```python
from build123d import *

# Parameters (mm, degrees)
F0_W     = 31.75
F0_H     = 44.45
F0_R     = 1.5875
F1_DEPTH = 25.4
F2_R     = 1.1303
F3_DEPTH = 6.35


with BuildPart() as f1:
    # F0 (on Front) → F1 (new body)
    with BuildSketch(Plane.XZ):
        with Locations((-15.875, 22.225)):
            Rectangle(F0_W, F0_H)
        with Locations((-25.4, 25.4)):
            Circle(F0_R, mode=Mode.SUBTRACT)
    extrude(amount=F1_DEPTH)

    # F2 (on Top) → F3 (cut)
    with BuildSketch(Plane.XY):
        with Locations((-21.166667, -12.7)):
            Circle(F2_R)
        with Locations((-10.583333, -12.7)):
            Circle(F2_R)
    extrude(amount=F3_DEPTH, mode=Mode.SUBTRACT)


solid = f1.part
```
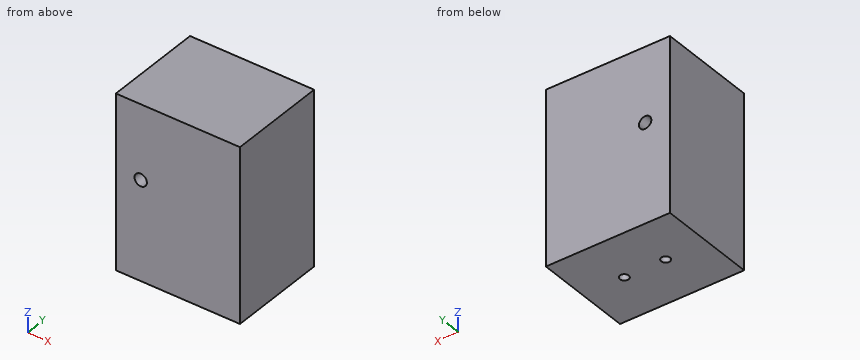
The model under review builds one solid part; all positions refer to its coordinate system, in mm. Round coordinates to 2 decimals unless told otherwise and drop trailing zeros. Loops run counter-clockwise (first coordinate to the right, second up) from the corner with the lowest first, then second, coordinate; pieces in that order, holes last. Notation, with made-up numbers: (-22, 21.25) - (30, 21.25) arc R28 cw to (30, 57.25) - close; hole circle Ø11 at (81.5, -20.5). An arc over 180 degrees is marked (long way). Use a Markdown table: item, result. Add a question column.
Q1. Add section C-C (x = -25.4). State the section outline as (y, z) points, plus the area to 3 significant figures.
Q2. Add section B-B (z = 25.4). State the section outline as (x, y) points.
Q3. Insertion check: pin 1 Ø1.1 at (x, y) = (-10.5, -12) entering from -Z; pin 2 Ø1.8 at (x, y) = (-21.17, -12.7) entering from -Z. Each pin has a flat end and moves straight along its axis. Give the tip position at first contact, or say it passes through.
Q4. For probe 1 along Z at (x, y) = (-25.4, -16.5); probe 2 along Z at (x, y) = (-10, -12); probe 3 along Z at (x, y) = (-26, -17.5), list the stretches that pass through material, from the lowest coordinate up.
Worked answers:
| question | item | result |
|---|---|---|
| 1 | outline | (-25.4, 0) - (0, 0) - (0, 23.81) - (-25.4, 23.81) - close; (-25.4, 26.99) - (0, 26.99) - (0, 44.45) - (-25.4, 44.45) - close |
| 1 | area | 1,050 mm² |
| 2 | outline | (-31.75, -25.4) - (-26.99, -25.4) - (-26.99, 0) - (-31.75, 0) - close; (-23.81, -25.4) - (0, -25.4) - (0, 0) - (-23.81, 0) - close |
| 3 | pin 1 | z = 0 |
| 3 | pin 2 | z = 6.35 |
| 4 | probe 1 | 0 to 23.81, 26.99 to 44.45 |
| 4 | probe 2 | 6.35 to 44.45 |
| 4 | probe 3 | 0 to 23.93, 26.87 to 44.45 |
